from build123d import *

# Parameters (mm, degrees)
SKETCH_1_W          = 56
SKETCH_1_H          = 65
EXTRUDE_1_DEPTH     = 7.8
SKETCH_3_R          = 4.75
CUT_EXTRUDE_2_DEPTH = 8.8
SKETCH_4_R          = 11
SKETCH_4_R_2        = 1.5
SKETCH_4_R_3        = 2.5
CUT_EXTRUDE_3_DEPTH = 8.8


with BuildPart() as part:
    # 草图1 → 凸台-拉伸1 (new body)
    with BuildSketch(Plane(origin=(0, 0, 0), x_dir=(1, 0, 0), z_dir=(0, 1, 0))):
        Rectangle(SKETCH_1_W, SKETCH_1_H)
    extrude(amount=EXTRUDE_1_DEPTH)

    # 草图3 → 切除-拉伸2 (cut, through all)
    with BuildSketch(Plane(origin=(0, 7.8, 0), x_dir=(1, 0, 0), z_dir=(0, 1, 0))):
        with Locations((-10, -23)):
            Circle(SKETCH_3_R)
        with Locations((10, -23)):
            Circle(SKETCH_3_R)
    extrude(amount=-CUT_EXTRUDE_2_DEPTH, mode=Mode.SUBTRACT)

    # 草图4 → 切除-拉伸3 (cut, through all)
    with BuildSketch(Plane(origin=(0, 7.8, 0), x_dir=(1, 0, 0), z_dir=(0, 1, 0))):
        with Locations((0, 3.5)):
            Circle(SKETCH_4_R)
        with Locations((-15.5, 19)):
            Circle(SKETCH_4_R_2)
        with Locations((15.5, 19)):
            Circle(SKETCH_4_R_2)
        with Locations((15.5, -12)):
            Circle(SKETCH_4_R_2)
        with Locations((-15.5, -12)):
            Circle(SKETCH_4_R_2)
        with Locations((-23.5, 27)):
            Circle(SKETCH_4_R_3)
        with Locations((23.5, 27)):
            Circle(SKETCH_4_R_3)
        with Locations((23.5, -20)):
            Circle(SKETCH_4_R_3)
        with Locations((-23.5, -20)):
            Circle(SKETCH_4_R_3)
    extrude(amount=-CUT_EXTRUDE_3_DEPTH, mode=Mode.SUBTRACT)


solid = part.part
Source: CAD feature listing. Evaluate the final solid. Frame: model axes, mm. Coordinates: 2 decimals unless noted, no trailing zeros. Order: outer loops, then holes, each group sorted by start corner. A loop starts at its lowest first (then second) coordinate and runs counter-clockwise, first axis right, second up. Notation, with made-up numbers: M 81.5,-24 L 131.5,-24 A14 ccw 131.5,-4 Z; hole C 69,48 d2. An arc over 180 degrees is marked long. Write each question's results on one line, items separated by ' | '. Start each with the question number.
1. Pin query (flat end, axial travel): pin 1 (4.5 mm diameter, centred on x = -23.5, z = -27, fed in from -Y). Return the tip coordinate at first contact, or that it passes through.
2. Section A-A, the plane x = 15.5. Return the cut outline in (y, z), then the cut area to 3 significant figures.
3. Section D-D, the plane z = 12. Return the cut outline in (x, y).
4. Section B-B, the plane z = -3.5. Return the cut outline in (x, y).
5. Section C-C, the plane y = 2.5. State how many separate pieces and enclosed holes the cut face has, then the cut area to 3 significant figures.
6. Material intervals for L1, parallel to Z at x = 23.5, y = 4.5; L2, parallel to X at y = 3.5, z = -19; L3, parallel to Z at x = 15.5, y = 2, sorted ascending.
Solution:
1) pin 1: through
2) outline: M 0,-32.5 L 7.8,-32.5 L 7.8,-20.5 L 0,-20.5 Z; M 0,-17.5 L 7.8,-17.5 L 7.8,10.5 L 0,10.5 Z; M 0,13.5 L 7.8,13.5 L 7.8,32.5 L 0,32.5 Z | area: 460 mm²
3) outline: M -28,0 L -17,0 L -17,7.8 L -28,7.8 Z; M -14,0 L 14,0 L 14,7.8 L -14,7.8 Z; M 17,0 L 28,0 L 28,7.8 L 17,7.8 Z
4) outline: M -28,0 L -11,0 L -11,7.8 L -28,7.8 Z; M 11,0 L 28,0 L 28,7.8 L 11,7.8 Z
5) separate pieces: 1 | enclosed holes: 11 | area: 3,010 mm²
6) L1: -32.5 to -29.5, -24.5 to 17.5, 22.5 to 32.5 | L2: -28 to -17, -14 to 14, 17 to 28 | L3: -32.5 to -20.5, -17.5 to 10.5, 13.5 to 32.5
